Read the model definition and answer for the solid it produces. Units are mm, in the model's axes. A direction names the side the tool comes from. Coordinates: 2 decimals unless noted, no trailing zeros. Write each loop counter-clockwise with the first axis right and the second up, starting at its lowest first coordinate (ties: lowest second). Pieces come first, ordered by that corner, then holes. Notation, with made-up numbers: M 63.25,-10 L 85.25,-10 A21 cw 85.25,17 Z; hole C 36,10.25 d11. An arc over 180 degrees is marked long. Write item = value, one per line.
from build123d import *

# Parameters (mm, degrees)
F1_DEPTH = 6.35
F2_W     = 2.774914
F2_H     = 7.584815
F3_DEPTH = 25.4


with BuildPart() as f1:
    # F0 (on Front) → F1 (new body)
    with BuildSketch(Plane.XZ):
        with BuildLine():
            ThreePointArc((12.063488, 0.970442), (10.987924, 12.058307), (0, 10.224426))
            ThreePointArc((0, 10.224426), (-10.883613, 12.136914), (-12.232943, 1.169236))
            Line((-12.232943, 1.169236), (-11.889853, 0.780254))
            Line((-11.889853, 0.780254), (0, -12.7))
            Line((0, -12.7), (12.063488, 0.970442))
        make_face()
    extrude(amount=F1_DEPTH)

    # F2 (on face) → F3 (cut)
    with BuildSketch(Plane.XZ.offset(6.35)):
        with Locations((-3.250018, 3.792407)):
            Rectangle(F2_W, F2_H)
        with Locations((3.250018, 3.792407)):
            Rectangle(F2_W, F2_H)
    extrude(amount=-F3_DEPTH, mode=Mode.SUBTRACT)


solid = f1.part
Item 1: Consider line 1 along X through (y, z) = (-2, 6); line 2 along X through (y, z) = (-5.25, 4); line 3 along Z through (x, y) = (2.25, -3.25). Determine where each line is inside the solid, lowest interval first. Write a range as from..to.
Worked answers:
line_1 = -13.97..-4.64, -1.86..1.86, 4.64..13.97
line_2 = -13.7..-4.64, -1.86..1.86, 4.64..13.7
line_3 = -10.15..0, 7.58..12.44
Item 2: For a pull along X with two mould halves and no side action, classify faces 1 (the face through (0, 0, 4)), 2 (the face through (-4.637, -3, 4)), 3 (the face through (5.95, -3.13, -5.96)) as released by +X, released by -X, zero draft, split by the parting line, or undercut.
Worked answers:
face_1 = zero draft
face_2 = undercut
face_3 = released by +X
Item 3: Find section B-B (z = -4). Determine the outline of the cut face in (x, y).
Worked answers:
outline = M -7.67,-6.35 L 7.68,-6.35 L 7.68,0 L -7.67,0 Z
Item 4: Flat-ended cylindrical pins translate along their axes: pin 1 (2 mm diameter, centred on y = -2.5, z = -8.5, fed in from +X); pin 2 (3 mm diameter, centred on x = -3.5, y = -4.5, fed in from +Z); pin 3 (3 mm diameter, centred on x = 4, y = -3, fed in from +Z). Find the tip coordinate at first contact, or state that the pin passes through.
Worked answers:
pin_1 = 4.59
pin_2 = 13.51
pin_3 = 13.58
Item 5: Find section A-A (y = -2.25). Determine the outline of the cut face in (x, z).
Worked answers:
outline = M -12.23,1.17 L -11.89,0.78 L 0,-12.7 L 12.06,0.97 A7.62 ccw long 0,10.22 A7.62 ccw long Z; hole M -4.64,0 L -1.86,0 L -1.86,7.58 L -4.64,7.58 Z; hole M 1.86,0 L 4.64,0 L 4.64,7.58 L 1.86,7.58 Z
Item 6: Which of the six approach directions +Z, -Z, +X, -X, +Y, -Y give full straight-line access (tool end or side, diameter ignored) to faces 4 (the face through (3, -3, 0)), 5 (the face through (0, -6.35, 4))?
Worked answers:
face_4 = +Y, -Y
face_5 = +Z, -Z, +X, -X, -Y
Item 7: Find section C-C (x = -6.35). Determine the outline of the cut face in (y, z), and give its area (3 significant figures).
Worked answers:
outline = M -6.35,-5.5 L 0,-5.5 L 0,13.63 L -6.35,13.63 Z
area = 121 mm²
